from build123d import *

# Parameters (mm, degrees)
SKETCH_1_R          = 3.1
SKETCH_1_R_2        = 2.1
EXTRUDE_1_DEPTH     = 4
SKETCH_2_W          = 35.5
SKETCH_2_H          = 4
EXTRUDE_2_DEPTH     = 4
CUT_EXTRUDE_1_DEPTH = 5
FILLET_1_R          = 3
FILLET_2_R          = 0.1


with BuildPart() as part:
    # 草图1 → 凸台-拉伸1 (new body)
    with BuildSketch(Plane(origin=(0, 0, 0), x_dir=(0, 0, -1), z_dir=(1, 0, 0))):
        with BuildLine():
            Line((-6.056426263, 3.50994315), (29, 64))
            Line((29, 64), (74, 64))
            Line((74, 64), (4.946141362, -4.95335095))
            ThreePointArc((4.946141362, -4.95335095), (-4.267905798, -5.548421406), (-6.056426263, 3.50994315))
        make_face()
        Circle(SKETCH_1_R, mode=Mode.SUBTRACT)
        with Locations((44, 60)):
            Circle(SKETCH_1_R_2, mode=Mode.SUBTRACT)
        with Locations((64, 60)):
            Circle(SKETCH_1_R_2, mode=Mode.SUBTRACT)
    extrude(amount=EXTRUDE_1_DEPTH)

    # 草图2 → 凸台-拉伸2 (add)
    with BuildSketch(Plane(origin=(4, 0, 0), x_dir=(0, 0, -1), z_dir=(1, 0, 0))):
        with Locations((56.25, 66)):
            Rectangle(SKETCH_2_W, SKETCH_2_H)
    extrude(amount=-EXTRUDE_2_DEPTH)

    # 草图3 → 切除-拉伸1 (cut, through all)
    with BuildSketch(Plane(origin=(4, 0, 0), x_dir=(0, 0, -1), z_dir=(1, 0, 0))):
        Polygon((74, 68), (68, 68), (68, 58.008732982), (74, 64), align=None)
    extrude(amount=-CUT_EXTRUDE_1_DEPTH, mode=Mode.SUBTRACT)

    # 圆角1
    fillet_1_edges = [part.edges().sort_by_distance(p)[0] for p in [
        (2, 68, -38.5),
        (2, 58.008732982, -68),
        (2, 68, -68),
        (2, 64, -29),
    ]]
    fillet(fillet_1_edges, radius=FILLET_1_R)

    # 圆角2
    fillet_2_edges = [part.edges().sort_by_distance(p)[0] for p in [
        (2, 64, -38.5),
    ]]
    fillet(fillet_2_edges, radius=FILLET_2_R)


solid = part.part
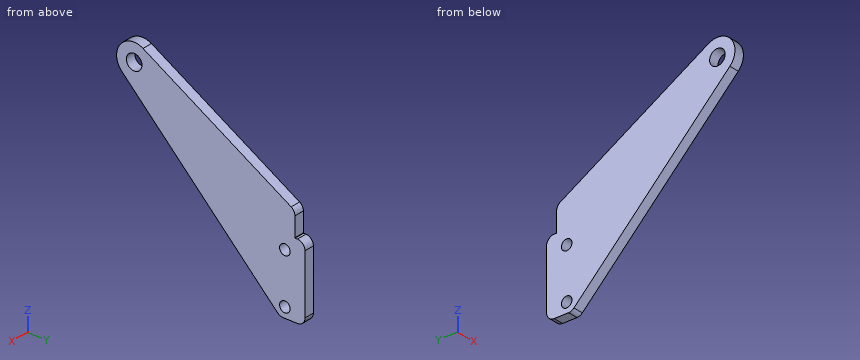
The listing builds one solid part. Answer for the finished solid, in the listing's coordinates (mm). Coordinates: 2 decimals unless noted, no trailing zeros. Write each loop counter-clockwise with the first axis right and the second up, starting at its lowest first coordinate (ties: lowest second). Pieces come first, ordered by that corner, then holes. Notation, with made-up numbers: M 20.25,-12.75 L 45.25,-12.75 A28 ccw 45.25,9.25 Z; hole C -4.75,-5.5 d4. An arc over 180 degrees is marked long. Use one line per item in the form item = value.
Item 1: Find the intervals of material crossed by probe 1 along Y at (x, z) = (2.2, 0); probe 2 along Y at (x, z) = (1.55, -44); probe 3 along Z at (x, y) = (0.5, 31.5), in increasing order.
Model answer:
probe_1 = -7 to -3.1, 3.1 to 13.96
probe_2 = 34.04 to 57.9, 62.1 to 68
probe_3 = -41.45 to -10.16
Item 2: Find section C-C, the plane y = 0. Give the vertices of the cut face in (x, z).
Model answer:
outline = M 0,-9.91 L 4,-9.91 L 4,-3.1 L 0,-3.1 Z; M 0,3.1 L 4,3.1 L 4,7 L 0,7 Z
Item 3: Find section B-B, the plane z = -44. Give the vertices of the cut face in (x, y), plus the area to 3 significant figures.
Model answer:
outline = M 0,34.04 L 4,34.04 L 4,57.9 L 0,57.9 Z; M 0,62.1 L 4,62.1 L 4,68 L 0,68 Z
area = 119 mm2
Item 4: Find section D-D, the plane y = 53. Give the vertices of the cut face in (x, z), plus the area to 3 significant figures.
Model answer:
outline = M 0,-62.98 L 4,-62.98 L 4,-22.63 L 0,-22.63 Z
area = 161 mm2
Item 5: Find section A-A, the plane x = 2.3. Give the vertices of the cut face in (y, z).
Model answer:
outline = M -4.95,-4.95 L 57.13,-67.12 A3 ccw 59.25,-68 L 65,-68 A3 ccw 68,-65 L 68,-41.5 A3 ccw 65,-38.5 L 64.1,-38.5 A0.1 cw 64,-38.4 L 64,-30.73 A3 ccw 62.5,-28.13 L 3.51,6.06 A7 ccw Z; hole C 0,0 d6.2; hole C 60,-64 d4.2; hole C 60,-44 d4.2
Item 6: Given P1, Ø2, axis at x = 2.5, z = -34.5, coming from the +Y side; P2, Ø0.5, axis at x = 1.5, y = 64.5, coming from the +Z side; P3, Ø4, axis at y = 60, z = -44, coming from the -X side, each flat-ended and moving along its own axis, determine where each tip first touches the part or whether it passes through.
Model answer:
P1 = 64
P2 = -38.5
P3 = through
